Can you work these out from the model? Positions are in its coordinate system, mm. A direction names the side the tool comes from. Round coordinates to 2 decimals unless told otherwise and drop trailing zeros. Write each loop counter-clockwise with the first axis right and the second up, starting at its lowest first coordinate (ties: lowest second). Pieces come first, ordered by that corner, then holes.
Q1. If we section it at D-D (z = 40): Please give me the cut outline in (x, y), plus the area to 3 significant figures.
Q2. We'd pull the mould along Z, two halves only. Please class faces 3 (the cylindrical face through (0.35, -4.49, 3.44)), 4 (the flat face through (-4.5, 0.1, 60)), 5 (the flat face through (-5, 0, 25)), 6 (the cylindrical face through (0.46, 4.51, 52.95)): +Z half, -Z half, draft (parallel to the pull), parting line (faces both ways), or undercut.
Q3. If we section it at A-A (z = -5): Please give me the cut outline in (x, y), plus the area to 3 significant figures.
Q4. If we section it at C-C (y = -3.25): Please give me the cut outline in (x, z), plus the area to 3 significant figures.
Q5. For faces 1 (the flat face through (4, 0, 25)), 2 (the cylindrical face through (0.46, -4.49, 52.95)), which set-ups out of +Z, -Z, +X, -X, +Y, -Y let a thin tool reach every point of the face, with its end or its side?
Q6. If we section it at B-B (x = 0): Give the number of separate pieces and of enclosed holes in the cut face, plus the area to 3 significant figures.
Q7. Please list where these lines run through material, in increasing order: line 1 along Z through (x, y) = (0, 4.5); line 2 along X through (y, z) = (1.5, 0.5); line 3 along Z through (x, y) = (-4.6, 0).
from build123d import *

# Parameters (mm, degrees)
SKETCH_1_W          = 10
SKETCH_1_H          = 10
SKETCH_1_W_2        = 8
SKETCH_1_H_2        = 8
EXTRUDE_1_DEPTH     = 60
SKETCH_3_R          = 2.1
SKETCH_3_R_2        = 1.6
CUT_EXTRUDE_1_DEPTH = 62.032778079
SKETCH_7_W          = 10
SKETCH_7_H          = 10
SKETCH_7_W_2        = 8
SKETCH_7_H_2        = 8
EXTRUDE_1_2_DEPTH   = 10
SKETCH_8_R          = 1.6
CUT_EXTRUDE_5_DEPTH = 62.032778079


with BuildPart() as part:
    # ｽｹｯﾁ1 → Extrude 1 (new body)
    with BuildSketch(Plane.XY):
        Rectangle(SKETCH_1_W, SKETCH_1_H)
        Rectangle(SKETCH_1_W_2, SKETCH_1_H_2, mode=Mode.SUBTRACT)
    extrude(amount=EXTRUDE_1_DEPTH)

    # ｽｹｯﾁ3 → ｶｯﾄ - 押し出し1 (cut, through all)
    with BuildSketch(Plane(origin=(0, 5, 0), x_dir=(1, 0, 0), z_dir=(0, 1, 0))):
        with Locations(Location((0, -55, 0), (0, 0, 180))):
            Circle(SKETCH_3_R)
        with Locations(Location((0, -29, 0), (0, 0, 180))):
            Circle(SKETCH_3_R)
        with Locations(Location((0, -5, 0), (0, 0, 180))):
            Circle(SKETCH_3_R_2)
    extrude(amount=-CUT_EXTRUDE_1_DEPTH, mode=Mode.SUBTRACT)

    # ｽｹｯﾁ7 → Extrude 1 2 (add)
    with BuildSketch(Plane(origin=(0, 0, 0), x_dir=(-1, 0, 0), z_dir=(0, 0, -1))):
        Rectangle(SKETCH_7_W, SKETCH_7_H)
        Rectangle(SKETCH_7_W_2, SKETCH_7_H_2, mode=Mode.SUBTRACT)
    extrude(amount=EXTRUDE_1_2_DEPTH)

    # ｽｹｯﾁ8 → ｶｯﾄ - 押し出し5 (cut, through all)
    with BuildSketch(Plane.ZY.offset(5)):
        with Locations(Location((-5, 0, 0), (0, 0, 270))):
            Circle(SKETCH_8_R)
    extrude(amount=-CUT_EXTRUDE_5_DEPTH, mode=Mode.SUBTRACT)


solid = part.part
A:
1. outline: (-5, -5) - (5, -5) - (5, 5) - (-5, 5) - close; hole (-4, -4) - (4, -4) - (4, 4) - (-4, 4) - close
1. area: 36.0 mm2
2. face 3: undercut
2. face 4: +Z half
2. face 5: draft
2. face 6: undercut
3. outline: (-5, -5) - (5, -5) - (5, -1.6) - (4, -1.6) - (4, -4) - (-4, -4) - (-4, -1.6) - (-5, -1.6) - close; (-5, 1.6) - (-4, 1.6) - (-4, 4) - (4, 4) - (4, 1.6) - (5, 1.6) - (5, 5) - (-5, 5) - close
3. area: 29.6 mm2
4. outline: (-5, -10) - (-4, -10) - (-4, 60) - (-5, 60) - close; (4, -10) - (5, -10) - (5, 60) - (4, 60) - close
4. area: 140 mm2
5. face 1: +Z, -Z
5. face 2: +Y, -Y
6. separate pieces: 8
6. enclosed holes: 0
6. area: 117 mm2
7. line 1: z = -10 to 3.4, 6.6 to 26.9, 31.1 to 52.9, 57.1 to 60
7. line 2: x = -5 to -4, 4 to 5
7. line 3: z = -10 to -6.6, -3.4 to 60
